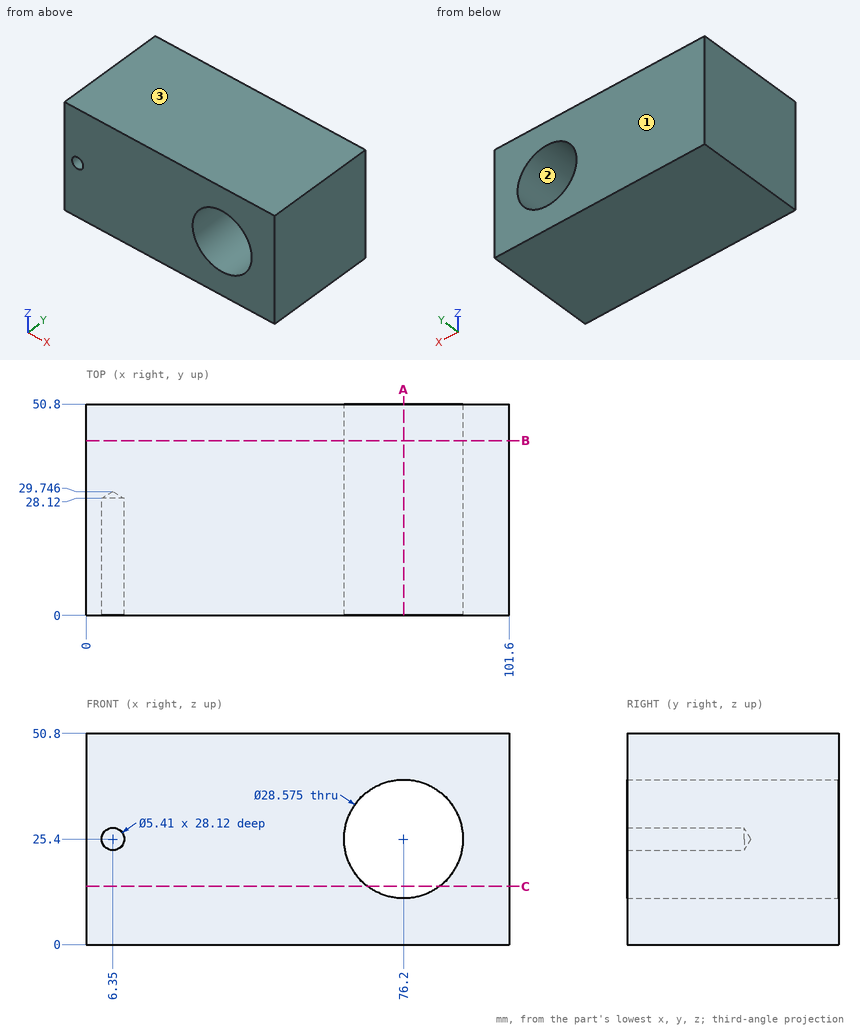
Source: three-view drawing plus pictorial views. Frame: mm from the lowest corner of the part. Give positions to 0.01 mm unless a question says otherwise; leave off trailing zeros. Write each loop counter-clockwise with the first axis right and the second up, starting at its lowest first coordinate (ties: lowest second). Pieces come first, ordered by that corner, then holes. Notation, with made-up numbers: (75.5, 55.25) - (129.5, 55.25) arc R36 cw to (129.5, 94.25) - close; hole circle Ø8 at (84.25, 3.5). An arc over 180 degrees is marked (long way). Write item = value, one per line. Start each with the question number.
Q1. Pin query (flat end, axial travel): pin 1 Ø3 at (x, z) = (6.35, 25.4) entering from -Y (1 decimal); pin 2 Ø17 at (x, z) = (76.2, 25.4) entering from -Y. Return the tip coordinate at first contact, or that it passes through.
Q2. Cut plane A-A, the plane x = 76.2. Return loops of the section in (y, z), then the cut area to 3 significant figures.
Q3. Material intervals for probe 1 along Z at (x, y) = (76.2, 36); probe 2 along Z at (x, y) = (6.35, 19.5) (1 decimal); probe 3 along X at (y, z) = (16.5, 25.4) (1 decimal), sorted ascending.
Q4. Cut plane B-B, the plane y = 42. Return loops of the section in (x, z) (1 decimal), then the cut area to 3 significant figures.
Q5. Cut plane C-C, the plane z = 14. Return loops of the section in (x, y).
Q6. Draft query along Z for the marked faces 1, 2 and 3. Return one class per face: +Z half, -Z half, draft (parallel to the pull), parting line (faces both ways), or undercut.
Computed values:
q1.pin_1 = 28.8
q1.pin_2 = through
q2.outline = (0, 0) - (50.8, 0) - (50.8, 11.11) - (0, 11.11) - close; (0, 39.69) - (50.8, 39.69) - (50.8, 50.8) - (0, 50.8) - close
q2.area = 1,130 mm²
q3.probe_1 = 0 to 11.11, 39.69 to 50.8
q3.probe_2 = 0 to 22.7, 28.1 to 50.8
q3.probe_3 = 0 to 3.6, 9.1 to 61.9, 90.5 to 101.6
q4.outline = (0, 0) - (101.6, 0) - (101.6, 50.8) - (0, 50.8) - close; hole circle Ø28.6 at (76.2, 25.4)
q4.area = 4,520 mm²
q5.outline = (0, 0) - (67.59, 0) - (67.59, 50.8) - (0, 50.8) - close; (84.81, 0) - (101.6, 0) - (101.6, 50.8) - (84.81, 50.8) - close
q6.face_1 = draft
q6.face_2 = undercut
q6.face_3 = +Z half
